Verification items for the finished model (mm, model axes). Face numbers are marked on the shaded views. A direction names the side the tool comes from. Give positions to 0.01 mm unless a question says otherwise; leave off trailing zeros. Write each loop counter-clockwise with the first axis right and the second up, starting at its lowest first coordinate (ties: lowest second). Pieces come first, ordered by that corner, then holes. Notation, with made-up numbers: M 2,84.5 L 15,84.5 A15 ccw 15,110.5 Z; hole C 84,-24.75 d5. An arc over 180 degrees is marked long. Write item = value, one per line.
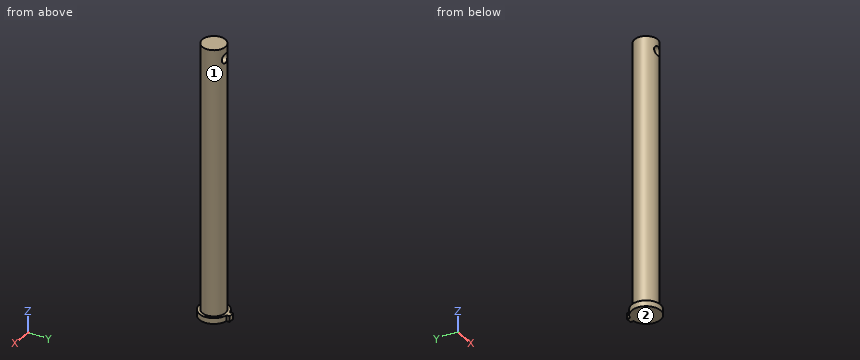
from build123d import *

# Parameters (mm, degrees)
SKETCH1_R                = 12.5
BOSS_EXTRUDE1_DEPTH      = 5
SKETCH3_R                = 10
BOSS_EXTRUDE2_DEPTH      = 230
CUT_EXTRUDE1_DEPTH       = 236.663955666
CUT_EXTRUDE1_DEPTH_BACK  = 236.663955666
SKETCH4_R                = 4
BOSS_EXTRUDE3_REACH      = 238.934
BOSS_EXTRUDE3_END_RADIUS = 12.5
SKETCH5_W                = 5
SKETCH5_H                = 5


with BuildPart() as part:
    # Sketch1 → Boss-Extrude1 (new body)
    with BuildSketch(Plane.XY):
        Circle(SKETCH1_R)
    extrude(amount=BOSS_EXTRUDE1_DEPTH)

    # Sketch3 → Boss-Extrude2 (add)
    with BuildSketch(Plane.XY.offset(5)):
        Circle(SKETCH3_R)
    extrude(amount=BOSS_EXTRUDE2_DEPTH)

    # Sketch4 → Cut-Extrude1 (cut, two sides: drawn at the far end of the back side and taken through both)
    with BuildSketch(Plane(origin=(0, 0, 0), x_dir=(1, 0, 0), z_dir=(0, 1, 0)).offset(-CUT_EXTRUDE1_DEPTH_BACK)):
        with Locations(Location((0, -225, 0), (0, 0, 270))):
            Circle(SKETCH4_R)
    extrude(amount=CUT_EXTRUDE1_DEPTH + CUT_EXTRUDE1_DEPTH_BACK, mode=Mode.SUBTRACT)

    # Boss-Extrude3: up to this cylinder (the profile starts outside it)
    boss_extrude3_end = Plane(origin=(0, 0, 2.5), z_dir=(0, 0, -1)) * Cylinder(BOSS_EXTRUDE3_END_RADIUS, 503.868, mode=Mode.PRIVATE)
    # Sketch5 → Boss-Extrude3 (add, up to the surface)
    with BuildSketch(Plane(origin=(0, 15, 0), x_dir=(1, 0, 0), z_dir=(0, 1, 0)), mode=Mode.PRIVATE) as boss_extrude3_sk1:
        with Locations((0, -2.5)):
            Rectangle(SKETCH5_W, SKETCH5_H)
    boss_extrude3_tool1 = extrude(boss_extrude3_sk1.sketch, amount=-BOSS_EXTRUDE3_REACH, mode=Mode.PRIVATE) - boss_extrude3_end
    add(boss_extrude3_tool1.solids().sort_by_distance((0, 15, 2.5))[0])


solid = part.part
1) Cross-section at B-B on y = 3. Record the boundary of the cut face in (x, z), plus the area to 3 significant figures.
From the geometry:
outline = M -12.13,0 L 12.13,0 L 12.13,5 L 9.54,5 L 9.54,235 L -9.54,235 L -9.54,5 L -12.13,5 Z; hole C 0,225 d8
area = 4,460 mm^2
2) Cross-section at A-A on x = 0. Record the boundary of the cut face in (y, z), plus the area to 3 significant figures.
From the geometry:
outline = M -12.5,0 L 15,0 L 15,5 L 10,5 L 10,221 L -10,221 L -10,5 L -12.5,5 Z; M -10,229 L 10,229 L 10,235 L -10,235 Z
area = 4,580 mm^2
3) Tool access check on the marked faces 1 and 2. Record the directions out of +Z, -Z, +X, -X, +Y, -Y that give a thin tool (end or side, any length) a straight path to the whole face; none if there is none.
From the geometry:
face_1 = +Z
face_2 = -Z, +X, -X, +Y, -Y
4) Cross-section at C-C on z = 225. Record the boundary of the cut face in (x, y).
From the geometry:
outline = M -4,-9.17 L -4,9.17 A10 ccw Z; M 4,-9.17 A10 ccw 4,9.17 Z
5) Material ranges on probe 1 along Z at (x, y) = (0, -1); probe 2 along X at (y, z) = (0.5, 24.5); probe 3 along X at (y, z) = (0.75, 225), recorded low to high. Write a range as from..to.
From the geometry:
probe_1 = 0..221, 229..235
probe_2 = -9.99..9.99
probe_3 = -9.97..-4, 4..9.97
6) Cross-section at D-D on z = 188. Record the boundary of the cut face in (x, y), plus the area to 3 significant figures.
From the geometry:
outline = C 0,0 d20
area = 314 mm^2
7) Depth check by flat-ended pin: P1, Ø1, axis at x = -8, z = 171.5, coming from the -Y side; P2, Ø6, axis at x = -1, z = 161, coming from the -Y side; P3, Ø10.5, axis at x = 0, z = 225, coming from the +Y side. Enter the tip coordinate at first touch or a pass-through.
From the geometry:
P1 = -6.61
P2 = -10
P3 = 10
